```python
from build123d import *

# Parameters (mm, degrees)
SKETCH1_W           = 190
SKETCH1_H           = 45
BOSS_EXTRUDE1_DEPTH = 10
SKETCH2_R           = 1.5
SKETCH2_R_2         = 12
SKETCH2_R_3         = 4
SKETCH2_R_4         = 2.75
SKETCH2_R_5         = 5
CUT_EXTRUDE1_DEPTH  = 10
CUT_EXTRUDE2_DEPTH  = 10
FILLET1_R           = 18


with BuildPart() as part:
    # Sketch1 → Boss-Extrude1 (new body)
    with BuildSketch(Plane(origin=(0, 0, 0), x_dir=(1, 0, 0), z_dir=(0, 1, 0))):
        Rectangle(SKETCH1_W, SKETCH1_H)
    extrude(amount=BOSS_EXTRUDE1_DEPTH)

    # Sketch2 → Cut-Extrude1 (cut)
    with BuildSketch(Plane(origin=(0, 10, 0), x_dir=(1, 0, 0), z_dir=(0, 1, 0))):
        with Locations(Location((-90.5, 15.5, 0), (0, 0, 270))):
            Circle(SKETCH2_R)
        with Locations(Location((-59.5, 15.5, 0), (0, 0, 270))):
            Circle(SKETCH2_R)
        with Locations(Location((-90.5, -15.5, 0), (0, 0, 270))):
            Circle(SKETCH2_R)
        with Locations(Location((-59.5, -15.5, 0), (0, 0, 270))):
            Circle(SKETCH2_R)
        with Locations(Location((-75, 0, 0), (0, 0, 270))):
            Circle(SKETCH2_R_2)
        with Locations(Location((-43, 0, 0), (0, 0, 270))):
            Circle(SKETCH2_R_3)
        with Locations(Location((-43, 16, 0), (0, 0, 270))):
            Circle(SKETCH2_R_4)
        with Locations(Location((-43, -16, 0), (0, 0, 90))):
            Circle(SKETCH2_R_4)
        with Locations(Location((77, 0, 0), (0, 0, 270))):
            Circle(SKETCH2_R_5)
    extrude(amount=-CUT_EXTRUDE1_DEPTH, mode=Mode.SUBTRACT)

    # Sketch3 → Cut-Extrude2 (cut)
    with BuildSketch(Plane(origin=(0, 10, 0), x_dir=(1, 0, 0), z_dir=(0, 1, 0))):
        Polygon((95, -22.5), (-5, -22.5), (95, -17.5), align=None)
        Polygon((-5, 22.5), (95, 17.5), (95, 22.5), align=None)
    extrude(amount=-CUT_EXTRUDE2_DEPTH, mode=Mode.SUBTRACT)

    # Fillet1
    fillet1_edges = [part.edges().sort_by_distance(p)[0] for p in [
        (95, 5, 17.5),
        (95, 5, -17.5),
    ]]
    fillet(fillet1_edges, radius=FILLET1_R)


solid = part.part
```
Here's how the part is built. I have some questions about the finished solid (model axes, mm). Give positions to 0.01 mm unless a question says otherwise; leave off trailing zeros. Write each loop counter-clockwise with the first axis right and the second up, starting at its lowest first coordinate (ties: lowest second). Pieces come first, ordered by that corner, then holes.
(1) If I drill on L1, parallel to X at y = 1.25, z = 0.5; L2, parallel to X at y = 3, z = -1.5; L3, parallel to Z at x = -68, y = 1, over which ranges is the centre line in solid material (lowest first)?
Output values:
L1: x = -95 to -86.99, -63.01 to -46.97, -39.03 to 72.03, 81.97 to 95
L2: x = -95 to -86.91, -63.09 to -46.71, -39.29 to 72.23, 81.77 to 94.96
L3: z = -22.5 to -9.75, 9.75 to 22.5
(2) Thinking about a two-plate mould opening in X: for faces 1 (the face through (-95, 5, 0)), 2 (the face through (-1, 10, 0)), 3 (the face through (-89.013, 5.07, 15.305)), 4 (the face through (35.869, 5.07, 20.457)), which applies, pulls with the +X half, pulls with the -X half, needs draft (parallel to the pull), parting line crosses it, or undercut?
Output values:
face 1: pulls with the -X half
face 2: needs draft
face 3: undercut
face 4: pulls with the +X half
(3) Imagine slicing it at C-C, the plane x = -75. Write out the boundary of the cut face in (y, z).
Output values:
outline: (0, -22.5) - (10, -22.5) - (10, -12) - (0, -12) - close; (0, 12) - (10, 12) - (10, 22.5) - (0, 22.5) - close
(4) Imagine slicing it at D-D, the plane x = 32. Write out the boundary of the cut face in (y, z).
Output values:
outline: (0, -20.65) - (10, -20.65) - (10, 20.65) - (0, 20.65) - close
(5) Imagine slicing it at B-B, the plane x = -43. Write out the boundary of the cut face in (y, z).
Output values:
outline: (0, -22.5) - (10, -22.5) - (10, -18.75) - (0, -18.75) - close; (0, -13.25) - (10, -13.25) - (10, -4) - (0, -4) - close; (0, 4) - (10, 4) - (10, 13.25) - (0, 13.25) - close; (0, 18.75) - (10, 18.75) - (10, 22.5) - (0, 22.5) - close
(6) Will these pins go through, and if not, where does the flat tip stop? pin 1 (4 mm diameter, centred on x = -59.5, z = 15.5, fed in from +Y); pin 2 (2 mm diameter, centred on y = 8.5, z = -6, fed in from +X); pin 3 (6 mm diameter, centred on x = 69, y = 1.5, fed in from +Z).
Output values:
pin 1: stops at y = 10
pin 2: stops at x = 94.4
pin 3: stops at z = 18.95
(7) Imagine slicing it at A-A, the plane y = 6. Count the separate pieces of the cut face and the enclosed holes in it, and give its area (3 significant figures).
Output values:
separate pieces: 1
enclosed holes: 9
area: 7,270 mm2
